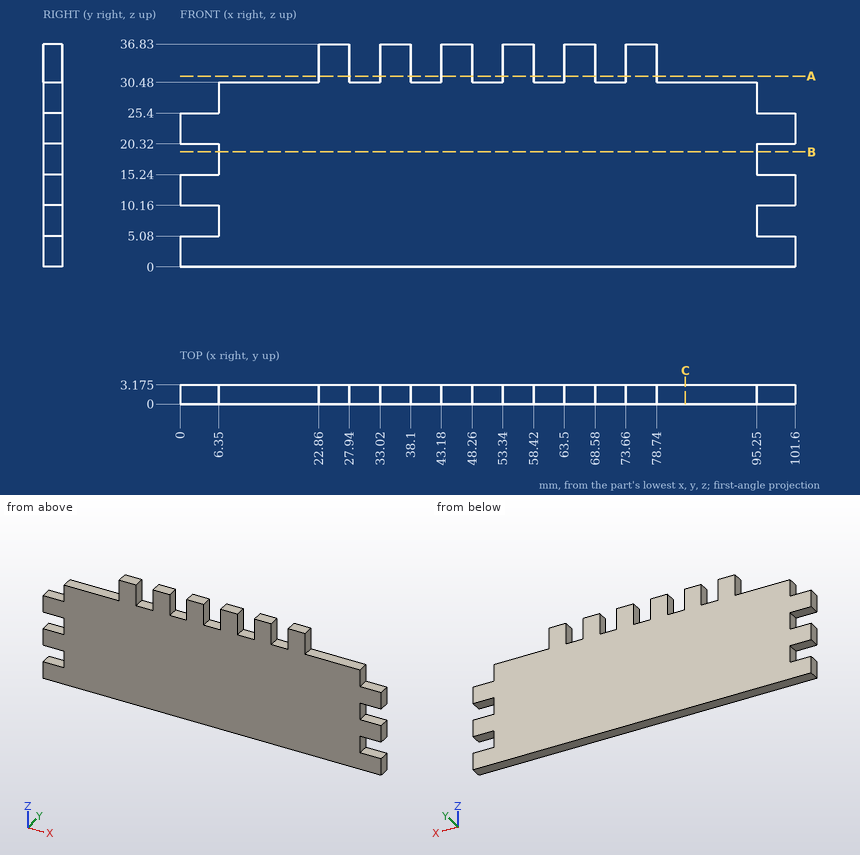
Study the drawing (mm; zero at the part's minimum x, y, z) and answer. Round coordinates to 2 decimals unless told otherwise and drop trailing zeros. Order: outer loops, then holes, each group sorted by start corner. A loop starts at its lowest first (then second) coordinate and runs counter-clockwise, first axis right, second up. Notation, with made-up numbers: (-27, 31.25) -> (10, 31.25) arc R18 cw to (10, 64.25) -> close; hole circle Ø6 at (-15.5, 28.5). An arc over 180 degrees is marked (long way). Answer as CSV lines item,"result". Start each with the question number.
(1) The part is cut by section C-C (x = 83.5). Determine the outline of the cut face in (y, z) (3 decimals).
(2) Flat-ended cylindrical pins translate along their axes: pin 1 Ø1 at (y, z) = (2, 34) entering from -X; pin 2 Ø1 at (y, z) = (2, 33) entering from +X; pin 3 Ø1.6 at (y, z) = (1, 7.5) entering from +X. Find the tip coordinate at first contact, or state that the pin passes through.
(3) Find the intervals of material crossed by probe 1 along X at (y, z) = (1.4, 34); probe 2 along X at (y, z) = (2.7, 7); probe 3 along Z at (x, y) = (39.5, 0.8), in increasing order. Write a range as from..to.
(4) The part is cut by section A-A (z = 31.5). Determine the outline of the cut face in (x, y) (3 decimals).
(5) The part is cut by section B-B (z = 19). Determine the outline of the cut face in (x, y) (3 decimals).
Evaluation:
1,outline,"(0, 0) -> (3.175, 0) -> (3.175, 30.48) -> (0, 30.48) -> close"
2,pin 1,"x = 22.86"
2,pin 2,"x = 78.74"
2,pin 3,"x = 95.25"
3,probe 1,"22.86..27.94, 33.02..38.1, 43.18..48.26, 53.34..58.42, 63.5..68.58, 73.66..78.74"
3,probe 2,"6.35..95.25"
3,probe 3,"0..30.48"
4,outline,"(22.86, 0) -> (27.94, 0) -> (27.94, 3.175) -> (22.86, 3.175) -> close; (33.02, 0) -> (38.1, 0) -> (38.1, 3.175) -> (33.02, 3.175) -> close; (43.18, 0) -> (48.26, 0) -> (48.26, 3.175) -> (43.18, 3.175) -> close; (53.34, 0) -> (58.42, 0) -> (58.42, 3.175) -> (53.34, 3.175) -> close; (63.5, 0) -> (68.58, 0) -> (68.58, 3.175) -> (63.5, 3.175) -> close; (73.66, 0) -> (78.74, 0) -> (78.74, 3.175) -> (73.66, 3.175) -> close"
5,outline,"(6.35, 0) -> (95.25, 0) -> (95.25, 3.175) -> (6.35, 3.175) -> close"
